Design review of the part built by this model. Coordinates are the model's own, in mm. Give positions to 0.01 mm unless a question says otherwise; leave off trailing zeros. Order: outer loops, then holes, each group sorted by start corner. A loop starts at its lowest first (then second) coordinate and runs counter-clockwise, first axis right, second up. Notation, with made-up numbers: M 67,53.25 L 99,53.25 A24 cw 99,92.25 Z; hole C -8,40.5 d3. An arc over 180 degrees is marked long. Put each result on its own line as item: value. Start each with the question number.
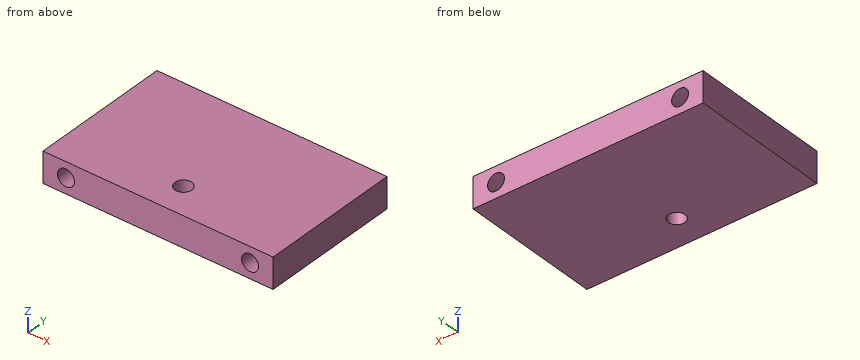
from build123d import *

# Parameters (mm, degrees)
SKETCH1_W           = 75
SKETCH1_H           = 10
SKETCH1_R           = 2.75
BOSS_EXTRUDE1_DEPTH = 46
SKETCH3_R           = 2.75
CUT_EXTRUDE1_DEPTH  = 45


with BuildPart() as part:
    # Sketch1 → Boss-Extrude1 (new body)
    with BuildSketch(Plane(origin=(0, 0, 0), x_dir=(1, 0, 0), z_dir=(0, 1, 0))):
        with Locations((37.5, 5)):
            Rectangle(SKETCH1_W, SKETCH1_H)
        with Locations(Location((7.5, 5, 0), (0, 0, 270))):
            Circle(SKETCH1_R, mode=Mode.SUBTRACT)
        with Locations(Location((67.5, 5, 0), (0, 0, 90))):
            Circle(SKETCH1_R, mode=Mode.SUBTRACT)
    extrude(amount=BOSS_EXTRUDE1_DEPTH)

    # Sketch3 → Cut-Extrude1 (cut)
    with BuildSketch(Plane.XY):
        with Locations((37.5, 10.25)):
            Circle(SKETCH3_R)
    extrude(amount=-CUT_EXTRUDE1_DEPTH, mode=Mode.SUBTRACT)


solid = part.part
1. Consider section D-D on y = 34. Give the boundary of the cut face in (x, z), then the cut area to 3 significant figures.
2. Consider section A-A on z = -5. Give the boundary of the cut face in (x, y), then the cut area to 3 significant figures.
3. Consider section B-B on y = 10.25. Give the boundary of the cut face in (x, z), then the cut area to 3 significant figures.
4. To check wall thickness, follow probe 1 along X at (y, z) = (23, -5); probe 2 along Y at (x, z) = (37.5, -6.5); probe 3 along X at (y, z) = (28, -4). State the ranges of each line that lie inside material, in increasing order.
5. Consider section C-C on x = 67.5. Give the boundary of the cut face in (y, z), then the cut area to 3 significant figures.
Returned:
1. outline: M 0,-10 L 75,-10 L 75,0 L 0,0 Z; hole C 7.5,-5 d5.5; hole C 67.5,-5 d5.5
1. area: 702 mm2
2. outline: M 0,0 L 4.75,0 L 4.75,46 L 0,46 Z; M 10.25,0 L 64.75,0 L 64.75,46 L 10.25,46 Z; M 70.25,0 L 75,0 L 75,46 L 70.25,46 Z; hole C 37.5,10.25 d5.5
2. area: 2,920 mm2
3. outline: M 0,-10 L 34.75,-10 L 34.75,0 L 0,0 Z; M 40.25,-10 L 75,-10 L 75,0 L 40.25,0 Z; hole C 7.5,-5 d5.5; hole C 67.5,-5 d5.5
3. area: 647 mm2
4. probe 1: x = 0 to 4.75, 10.25 to 64.75, 70.25 to 75
4. probe 2: y = 0 to 7.5, 13 to 46
4. probe 3: x = 0 to 4.94, 10.06 to 64.94, 70.06 to 75
5. outline: M 0,-10 L 46,-10 L 46,-7.75 L 0,-7.75 Z; M 0,-2.25 L 46,-2.25 L 46,0 L 0,0 Z
5. area: 207 mm2
